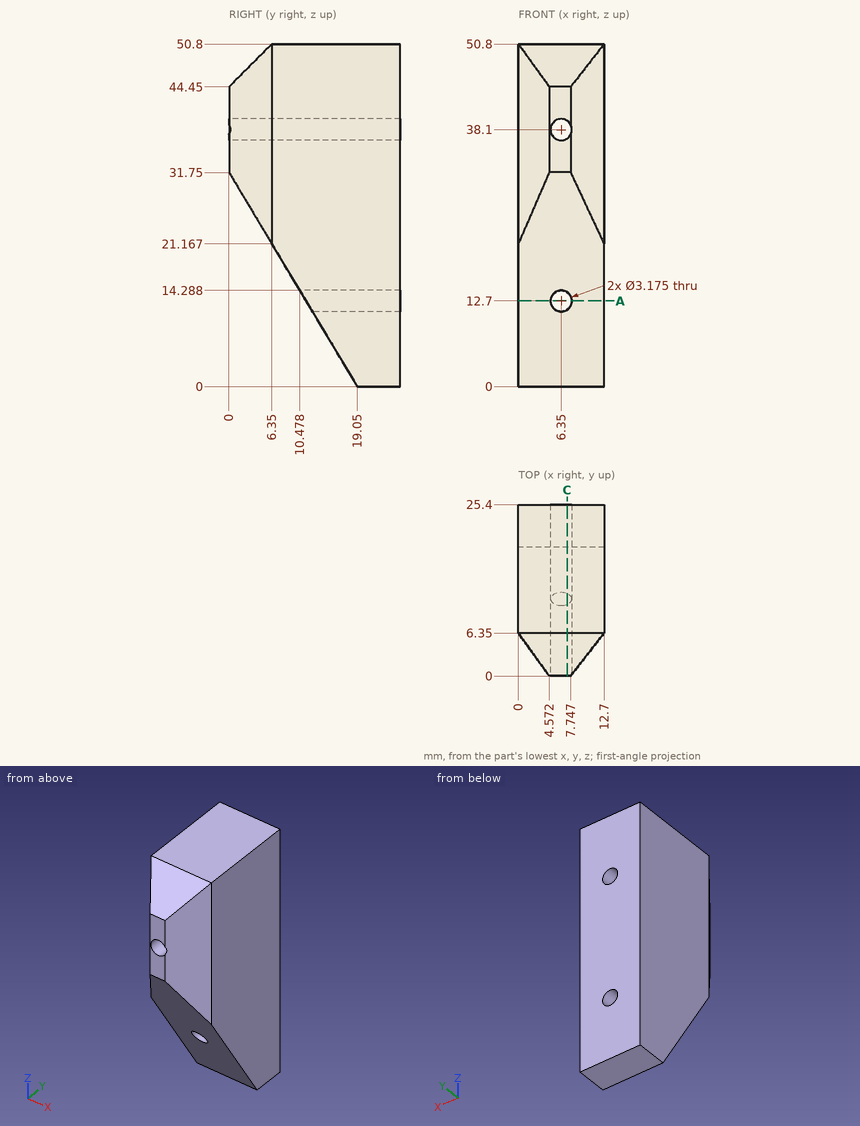
The drawing under review shows one solid part. Ordinate dimensions are in mm from its lowest x, y, z. Give positions to 0.01 mm unless a question says otherwise; leave off trailing zeros. Order: outer loops, then holes, each group sorted by start corner. A loop starts at its lowest first (then second) coordinate and runs counter-clockwise, first axis right, second up. Notation, with made-up numbers: M -21,-11 L 30,-11 A24 ccw 30,2 Z; hole C -18,53.25 d8. An arc over 180 degrees is marked long. Answer in a Markdown table with one row per item. Add a question column.
1. Add section A-A on z = 12.7. State the section outline as (x, y) points, plus the area to 3 significant figures.
2. Add section C-C on x = 7.25. Count the separate pieces of the cut face and the enclosed holes in it, plus the area to 3 significant figures.
3. For pin 1 Ø3 at (y, z) = (3, 27) entering from -X; pin 2 Ø4 at (x, z) = (6.35, 12.7) entering from -Y, all flat-tipped, find the tip position at first contact; note any pin that passes through.
4. To check wall thickness, follow line 1 along Z through (x, y) = (6.35, 19.25); line 2 along Z through (x, y) = (6.25, 14) (1 decimal); line 3 along X through (y, z) = (22.75, 12.7). State the ranges of each line that lie inside material, in increasing order.
The answers:
| question | item | result |
|---|---|---|
| 1 | outline | M 0,11.43 L 4.76,11.43 L 4.76,25.4 L 0,25.4 Z; M 7.94,11.43 L 12.7,11.43 L 12.7,25.4 L 7.94,25.4 Z |
| 1 | area | 133 mm2 |
| 2 | separate pieces | 3 |
| 2 | enclosed holes | 0 |
| 2 | area | 865 mm2 |
| 3 | pin 1 | x = 1.33 |
| 3 | pin 2 | y = 10.23 |
| 4 | line 1 | 0 to 11.11, 14.29 to 36.51, 39.69 to 50.8 |
| 4 | line 2 | 8.4 to 11.1, 14.3 to 36.5, 39.7 to 50.8 |
| 4 | line 3 | 0 to 4.76, 7.94 to 12.7 |
